Check sheet for the modelled part. Datum: model origin and axes. Units: mm. A direction names the side the tool comes from. Coordinates: 2 decimals unless noted, no trailing zeros. Loops run counter-clockwise (first coordinate to the right, second up) from the corner with the lowest first, then second, coordinate; pieces in that order, holes last. Notation, with made-up numbers: (-22.5, 67.25) - (21.5, 67.25) arc R30 ccw to (21.5, 99.25) - close; hole circle Ø4 at (-16, 44). An arc over 180 degrees is marked (long way). Write each question's results on one line, items separated by ' | '. Start each with the question number.
1. Gauge pin test, flat end, axial feed: P1, Ø4, axis at x = 0, y = 25, coming from the -Z side. Record the tip position at first contact, or that the pin passes through.
2. Cross-section at C-C (z = 1.5). Record the cut outline in (x, y).
3. Cross-section at A-A (y = -2.5). Record the cut outline in (x, z) (3 decimals), and give its area (3 significant figures).
4. Thickness scan on line 1 (X direction, y = -25, z = 0.9); line 2 (Y direction, x = -44.5, z = 1.3); line 3 (X direction, y = 1, z = 2.7). Record the ranges inside material, lowest first. Write a range as [from, to].
5. Draft check along X on faces 1 (the face through (17.5, -16.5, 1.6)), 2 (the face through (19.99, 37.15, 1.61)), 3 (the face through (-29, 1, 0)). Enter one of: released by +X, released by -X, zero draft, split by the parting line, or undercut.
6. Cross-section at D-D (y = 25). Record the cut outline in (x, z) (3 decimals).
7. Cross-section at B-B (x = -27.5). Record the cut outline in (y, z) (3 decimals).
8. Tool access check on faces 4 (the face through (-22, 25, 2)), 5 (the face through (-29, 40, 2)). Record the directions out of +Z, -Z, +X, -X, +Y, -Y that give a thin tool (end or side, any length) a straight path to the whole face; none if there is none.
```python
from build123d import *

# Parameters (mm, degrees)
SKETCH1_W           = 102.5
SKETCH1_H           = 80
SKETCH1_R           = 2.5
BOSS_EXTRUDE1_DEPTH = 3.175
FILLET1_R           = 10


with BuildPart() as part:
    # Sketch1 → Boss-Extrude1 (new body)
    with BuildSketch(Plane.XY):
        with Locations((-28.25, 0)):
            Rectangle(SKETCH1_W, SKETCH1_H)
        with Locations((0, 25)):
            Circle(SKETCH1_R, mode=Mode.SUBTRACT)
        with Locations(Location((0, -25, 0), (0, 0, 180))):
            Circle(SKETCH1_R, mode=Mode.SUBTRACT)
        with BuildLine():
            Line((-64.5, -27.5), (-24.5, -27.5))
            ThreePointArc((-24.5, -27.5), (-22, -25), (-24.5, -22.5))
            Line((-24.5, -22.5), (-64.5, -22.5))
            ThreePointArc((-64.5, -22.5), (-67, -25), (-64.5, -27.5))
        make_face(mode=Mode.SUBTRACT)
        with BuildLine():
            Line((-64.5, 27.5), (-24.5, 27.5))
            ThreePointArc((-24.5, 27.5), (-22, 25), (-24.5, 22.5))
            Line((-24.5, 22.5), (-64.5, 22.5))
            ThreePointArc((-64.5, 22.5), (-67, 25), (-64.5, 27.5))
        make_face(mode=Mode.SUBTRACT)
        with BuildLine():
            Line((19, 15), (19, -15))
            ThreePointArc((19, -15), (17.5, -16.5), (16, -15))
            Line((16, -15), (16, 15))
            ThreePointArc((16, 15), (17.5, 16.5), (19, 15))
        make_face(mode=Mode.SUBTRACT)
    extrude(amount=BOSS_EXTRUDE1_DEPTH)

    # Fillet1
    fillet1_edges = [part.edges().sort_by_distance(p)[0] for p in [
        (23, -40, 1.5875),
        (-79.5, -40, 1.5875),
        (-79.5, 40, 1.5875),
        (23, 40, 1.5875),
    ]]
    fillet(fillet1_edges, radius=FILLET1_R)


solid = part.part
```
Established:
1) P1: through
2) outline: (-79.5, -30) arc R10 ccw to (-69.5, -40) - (13, -40) arc R10 ccw to (23, -30) - (23, 30) arc R10 ccw to (13, 40) - (-69.5, 40) arc R10 ccw to (-79.5, 30) - close; hole (-64.5, -27.5) - (-24.5, -27.5) arc R2.5 ccw to (-24.5, -22.5) - (-64.5, -22.5) arc R2.5 ccw to start; hole (-64.5, 22.5) - (-24.5, 22.5) arc R2.5 ccw to (-24.5, 27.5) - (-64.5, 27.5) arc R2.5 ccw to start; hole circle Ø5 at (0, -25); hole circle Ø5 at (0, 25); hole (16, -15) arc R1.5 ccw to (19, -15) - (19, 15) arc R1.5 ccw to (16, 15) - close
3) outline: (-79.5, 0) - (16, 0) - (16, 3.175) - (-79.5, 3.175) - close; (19, 0) - (23, 0) - (23, 3.175) - (19, 3.175) - close | area: 316 mm^2
4) line 1: [-79.5, -67], [-22, -2.5], [2.5, 23] | line 2: [-40, -27.5], [-22.5, 22.5], [27.5, 40] | line 3: [-79.5, 16], [19, 23]
5) face 1: undercut | face 2: released by +X | face 3: zero draft
6) outline: (-79.5, 0) - (-67, 0) - (-67, 3.175) - (-79.5, 3.175) - close; (-22, 0) - (-2.5, 0) - (-2.5, 3.175) - (-22, 3.175) - close; (2.5, 0) - (23, 0) - (23, 3.175) - (2.5, 3.175) - close
7) outline: (-40, 0) - (-27.5, 0) - (-27.5, 3.175) - (-40, 3.175) - close; (-22.5, 0) - (22.5, 0) - (22.5, 3.175) - (-22.5, 3.175) - close; (27.5, 0) - (40, 0) - (40, 3.175) - (27.5, 3.175) - close
8) face 4: +Z, -Z | face 5: +Z, -Z, +X, -X, +Y
